Could you check a few things on this model? Use its own coordinates, in mm. Face numbers are marked on the shaded views. A direction names the side the tool comes from. Coordinates: 2 decimals unless noted, no trailing zeros. Order: outer loops, then holes, each group sorted by start corner. A loop starts at its lowest first (then second) coordinate and runs counter-clockwise, first axis right, second up. Notation, with made-up numbers: (28, 45.25) -> (62, 45.25) arc R20 cw to (62, 80.25) -> close; hole circle Ø8 at (-21, 44.25). An arc over 180 degrees is marked (long way). Use a Markdown table: item, result. Add a question column.
1) Will these pins go through, and if not, where does the flat tip stop? pin 1 Ø4 at (x, y) = (124.5, 52.5) entering from +Z; pin 2 Ø10 at (x, y) = (-81, 8.5) entering from -Z; pin 3 Ø10 at (x, y) = (-50.5, 61.5) entering from -Z.
2) If I drill on L1, parallel to Z at x = 43, y = 68; L2, parallel to Y at x = -116, z = 123.5; L3, parallel to X at y = 55, z = 85.5, over which ranges is the centre line in solid material (lowest first)? Write a range as [from, to].
3) Thinking about a two-plate mould opening in X: for the marked faces 1, 2 and 3, which applies, +X half, -X half, draft (parallel to the pull), parting line (faces both ways), or undercut?
4) If we section it at B-B (z = 57): Write out the boundary of the cut face in (x, y).
5) If we section it at A-A (y = 31.5): Write out the boundary of the cut face in (x, z), plus the area to 3 significant figures.
6) If we section it at D-D (z = 145.5): Write out the boundary of the cut face in (x, y), plus the area to 3 significant figures.
7) If we section it at C-C (x = 22.5): Write out the boundary of the cut face in (y, z).
8) Which directions (+Z, -Z, +X, -X, +Y, -Y) give clear straight access to the entire face, cutting with the end or side of a thin tool? Please do the marked faces 4 and 5.
```python
from build123d import *

# Parameters (mm, degrees)
BOSS_EXTRUDE1_DEPTH = 80
BOSS_EXTRUDE2_DEPTH = 5


with BuildPart() as part:
    # Sketch1 → Boss-Extrude1 (new body)
    with BuildSketch(Plane(origin=(0, 0, 0), x_dir=(1, 0, 0), z_dir=(0, 1, 0))):
        with BuildLine():
            Line((-68.405029852, -41.523820038), (-156.962867052, -97.747709945))
            ThreePointArc((-156.962867052, -97.747709945), (13.312357604, -184.430847657), (169.373640638, -74.192494834))
            Line((169.373640638, -74.192494834), (66.212991348, -44.936794682))
            ThreePointArc((66.212991348, -44.936794682), (-2.028141312, -79.996014791), (-68.405029852, -41.523820038))
        make_face()
        with BuildLine():
            Line((-34.725471354, -75.235438156), (-63.687790654, -169.483352526))
            ThreePointArc((-63.687790654, -169.483352526), (-113.842495993, -140.785750585), (-152.401202956, -97.747709945))
            Line((-152.401202956, -97.747709945), (-68.405029852, -46.765173005))
            ThreePointArc((-68.405029852, -46.765173005), (-53.494056391, -63.282030989), (-34.725471354, -75.235438156))
        make_face(mode=Mode.SUBTRACT)
        with BuildLine():
            Line((30.443645827, -77.067593345), (69.946567205, -166.997662253))
            ThreePointArc((69.946567205, -166.997662253), (4.833688489, -180.989991208), (-60.933223363, -170.493060716))
            Line((-60.933223363, -170.493060716), (-32.261228696, -76.324587377))
            ThreePointArc((-32.261228696, -76.324587377), (-0.981792411, -82.856898318), (30.443645827, -77.067593345))
        make_face(mode=Mode.SUBTRACT)
        with BuildLine():
            Line((67.248014437, -48.414192851), (164.278182262, -76.114520917))
            ThreePointArc((164.278182262, -76.114520917), (126.518982101, -129.513275883), (72.251766234, -166.013323977))
            Line((72.251766234, -166.013323977), (33.067262274, -75.978850221))
            ThreePointArc((33.067262274, -75.978850221), (52.01674028, -64.50184684), (67.248014437, -48.414192851))
        make_face(mode=Mode.SUBTRACT)
    extrude(amount=BOSS_EXTRUDE1_DEPTH)

    # Sketch4 → Boss-Extrude2 (add)
    with BuildSketch(Plane.XZ):
        with BuildLine():
            Line((-156.962867052, 97.747709945), (-68.405029852, 41.523820038))
            ThreePointArc((-68.405029852, 41.523820038), (-2.028141312, 79.996014791), (66.212991348, 44.936794682))
            Line((66.212991348, 44.936794682), (169.373640638, 74.192494834))
            ThreePointArc((169.373640638, 74.192494834), (13.312357604, 184.430847657), (-156.962867052, 97.747709945))
        make_face()
    extrude(amount=-BOSS_EXTRUDE2_DEPTH)


solid = part.part
```
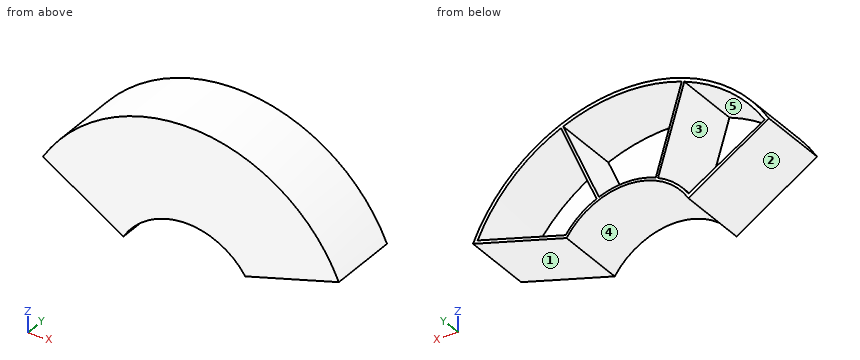
Answer sheet:
| question | item | result |
|---|---|---|
| 1 | pin 1 | z = 138.51 |
| 1 | pin 2 | z = 46.35 |
| 1 | pin 3 | z = 57.65 |
| 2 | L1 | [67.49, 70.83], [98.8, 105.65], [175.87, 179.84] |
| 2 | L2 | [0, 5] |
| 2 | L3 | [-137.67, -132.22], [-37.88, -35.05], [34.15, 37.21], [159.59, 163.96] |
| 3 | face 1 | +X half |
| 3 | face 2 | -X half |
| 3 | face 3 | undercut |
| 4 | outline | (-92.78, 0) -> (-56.16, 0) -> (-56.16, 80) -> (-60.14, 80) -> (-60.14, 5) -> (-85.27, 5) -> (-85.27, 80) -> (-92.78, 80) -> close; (56.16, 0) -> (108.75, 0) -> (108.75, 80) -> (97.32, 80) -> (97.32, 5) -> (60.14, 5) -> (60.14, 80) -> (56.16, 80) -> close |
| 5 | outline | (-156.96, 97.75) -> (-68.41, 41.52) arc R80.02 cw to (66.21, 44.94) -> (169.37, 74.19) arc R184.91 ccw to start; hole (-152.4, 97.75) -> (-68.41, 46.77) arc R82.86 cw to (-34.73, 75.24) -> (-63.69, 169.48) arc R181.05 ccw to start; hole (-60.93, 170.49) -> (-32.26, 76.32) arc R82.86 cw to (30.44, 77.07) -> (69.95, 167) arc R181.05 ccw to start; hole (33.07, 75.98) arc R82.86 cw to (67.25, 48.41) -> (164.28, 76.11) arc R181.05 ccw to (72.25, 166.01) -> close |
| 5 | area | 3,190 mm2 |
| 6 | outline | (-114.11, 0) -> (114.11, 0) -> (114.11, 80) -> (107.75, 80) -> (107.75, 5) -> (63.32, 5) -> (63.32, 80) -> (60.5, 80) -> (60.5, 5) -> (-53.32, 5) -> (-53.32, 80) -> (-56.32, 80) -> (-56.32, 5) -> (-107.75, 5) -> (-107.75, 80) -> (-114.11, 80) -> close |
| 6 | area | 2,530 mm2 |
| 7 | outline | (0, 76.79) -> (80, 76.79) -> (80, 79.75) -> (5, 79.75) -> (5, 179.65) -> (80, 179.65) -> (80, 183.54) -> (0, 183.54) -> close |
| 8 | face 4 | -Z, +Y, -Y |
| 8 | face 5 | +Y |
